Drawing for the job (mm, zero at the part's lowest x, y, z). A direction names the side the tool comes from. Round coordinates to 2 decimals unless told otherwise and drop trailing zeros. Write each loop counter-clockwise with the first axis right and the second up, starting at its lowest first coordinate (ties: lowest second). Pieces come first, ordered by that corner, then holes. Notation, with made-up numbers: (63, 40.5) -> (94, 40.5) arc R24 cw to (94, 69.5) -> close; hole circle Ø4 at (-38, 87). An arc over 180 degrees is marked (long way). One line per question, with ' | ' between items.
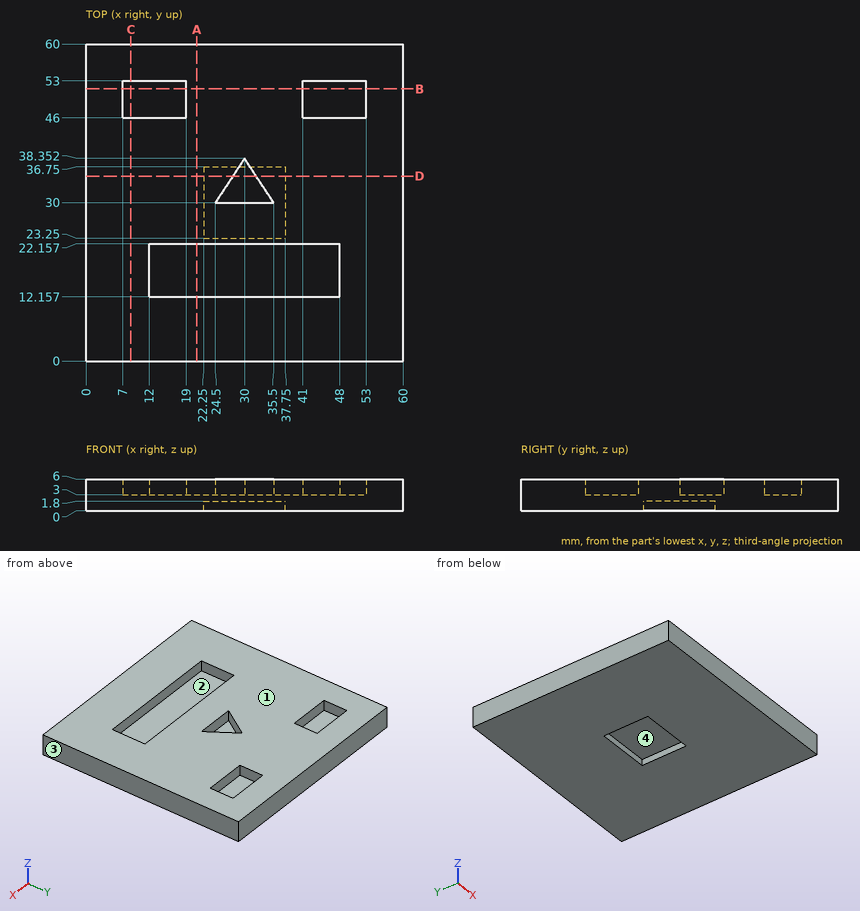
(1) 3-axis set-ups, long thin cutter, end or side, ignore diameter. For the marked faces 3 and 4: which of +Z, -Z, +X, -X, +Y, -Y reach the whole face in a straight line?
Calculated:
face 3: +Z, -Z, +X, +Y, -Y | face 4: -Z
(2) Slice it at A-A (x = 21). Write the cut outline in (y, z).
Calculated:
outline: (0, 0) -> (60, 0) -> (60, 6) -> (22.16, 6) -> (22.16, 3) -> (12.16, 3) -> (12.16, 6) -> (0, 6) -> close
(3) Slice it at B-B (y = 51.5). Write the cut outline in (x, z), then the cut area to 3 significant figures.
Calculated:
outline: (0, 0) -> (60, 0) -> (60, 6) -> (53, 6) -> (53, 3) -> (41, 3) -> (41, 6) -> (19, 6) -> (19, 3) -> (7, 3) -> (7, 6) -> (0, 6) -> close | area: 288 mm2
(4) Mould opens along Y. For the marked faces 1 and 2 say: pulls with the +Y half, pulls with the -Y half, needs draft (parallel to the pull), parting line crosses it, or undercut.
Calculated:
face 1: needs draft | face 2: undercut
(5) Slice it at D-D (y = 35). Write the cut outline in (x, z).
Calculated:
outline: (0, 0) -> (22.25, 0) -> (22.25, 1.8) -> (37.75, 1.8) -> (37.75, 0) -> (60, 0) -> (60, 6) -> (32.21, 6) -> (32.21, 3) -> (27.79, 3) -> (27.79, 6) -> (0, 6) -> close
(6) Slice it at C-C (x = 8.5). Write the cut outline in (y, z).
Calculated:
outline: (0, 0) -> (60, 0) -> (60, 6) -> (53, 6) -> (53, 3) -> (46, 3) -> (46, 6) -> (0, 6) -> close
(7) Wall check: line 1 (Y direction, x = 14, z = 3.15); line 2 (X direction, y = 30, z = 0.6); line 3 (X direction, y = 19.5, z = 5.2). Give the ranges that are in metal, low to high. Write a range as from..to.
Calculated:
line 1: 0..12.16, 22.16..46, 53..60 | line 2: 0..22.25, 37.75..60 | line 3: 0..12, 48..60
(8) Drop a flat-ended pin along its axis: pin 1 (2 mm diameter, centred on x = 46.5, y = 50.5, fed in from +Z). Give the stop position or say it passes through.
Calculated:
pin 1: z = 3
